Job drawing, mm, ordinate dimensions from the low corner. One solid piece. A direction names the side the tool comes from. Round coordinates to 2 decimals unless told otherwise and drop trailing zeros. Write each loop counter-clockwise with the first axis right and the second up, starting at its lowest first coordinate (ties: lowest second). Pieces come first, ordered by that corner, then holes. Notation, with made-up numbers: (47.25, 13) -> (52.25, 13) arc R23 ccw to (52.25, 42) -> close; hole circle Ø5 at (-2.75, -11). An arc over 180 degrees is marked (long way). Use CSV: the item, a comma, the result in double quotes. Start each with the question number.
(1) Saw through at B-B (x = 11). Give the cut face in (y, z), plus the area to 3 significant figures.
(2) Which spindle directions (+Z, -Z, +X, -X, +Y, -Y) get a long thin tool onto all of the face, cutting with end or side? Do the marked faces 1, 2 and 3. Say none if no direction does.
(3) Saw through at A-A (z = 5). Give the cut face in (x, y).
(4) Probe line 1 (Z direction, x = 11, y = 2.4); line 2 (X direction, y = 14.5, z = 4.75); line 3 (Y direction, x = 1.75, z = 4.75). List the from-to ranges inside material, lowest first. Write a range as [from, to].
(5) Saw through at D-D (x = 2.5). Give the cut face in (y, z).
(6) Drop flat-ended pins along their axis: pin 1 (2.5 mm diameter, centred on y = 11.5, z = 3.5, fed in from +X); pin 2 (3 mm diameter, centred on y = 15.5, z = 6.5, fed in from -X); pin 3 (1.5 mm diameter, centred on x = 18, z = 5.5, fed in from +Y); pin 4 (2.5 mm diameter, centred on y = 18.5, z = 7.5, fed in from +X). Give the stop position or say it passes through.
(7) Two-plate mould, pull along Y, no slides. Class the marked faces 4, 5 and 6: released by +Y, released by -Y, zero draft, split by the parting line, or undercut.
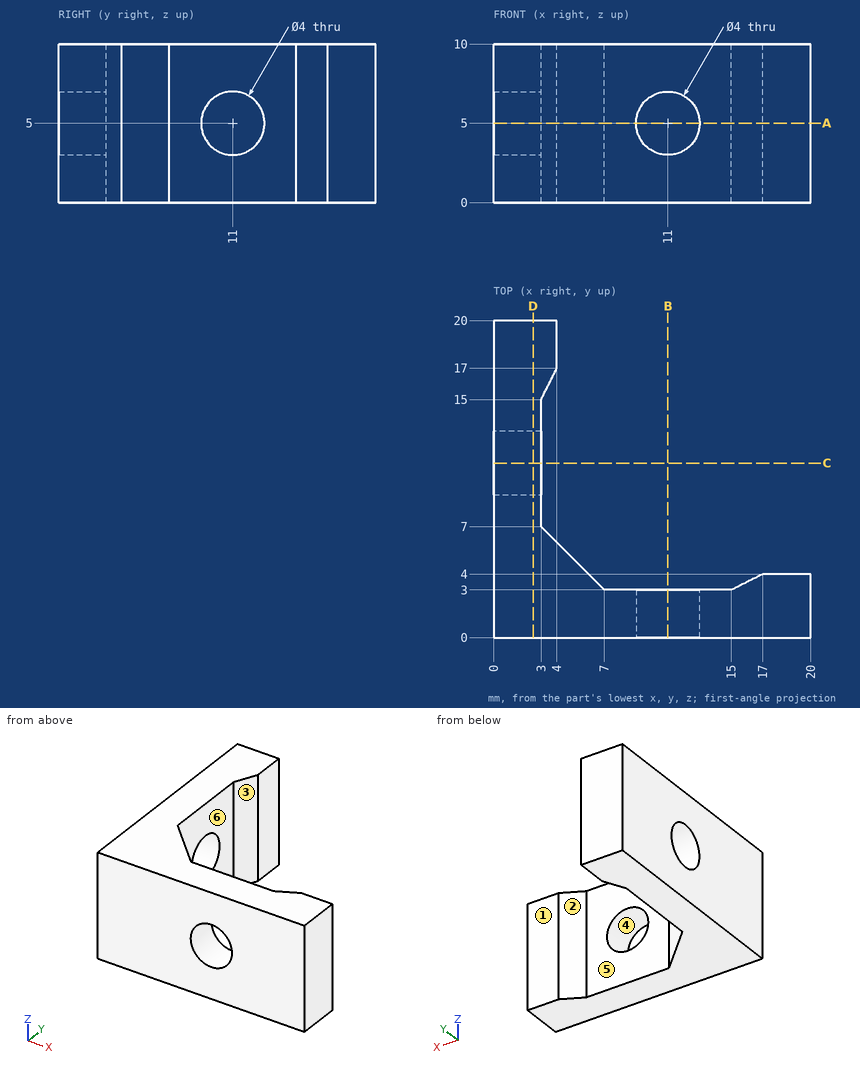
Answers:
1,outline,"(0, 0) -> (3, 0) -> (3, 3) -> (0, 3) -> close; (0, 7) -> (3, 7) -> (3, 10) -> (0, 10) -> close"
1,area,"18.0 mm²"
2,face 1,"+Z, -Z, +X, +Y"
2,face 2,"+Z, -Z, +Y"
2,face 3,"+Z, -Z, +X"
3,outline,"(0, 0) -> (9, 0) -> (9, 3) -> (7, 3) -> (3, 7) -> (3, 9) -> (0, 9) -> close; (0, 13) -> (3, 13) -> (3, 15) -> (4, 17) -> (4, 20) -> (0, 20) -> close; (13, 0) -> (20, 0) -> (20, 4) -> (17, 4) -> (15, 3) -> (13, 3) -> close"
4,line 1,"z = [0, 3], [7, 10]"
4,line 2,"x = [0, 3]"
4,line 3,"y = [0, 9.02], [12.98, 20]"
5,outline,"(0, 0) -> (20, 0) -> (20, 10) -> (0, 10) -> close; hole circle Ø4 at (11, 5)"
6,pin 1,"stops at x = 3"
6,pin 2,"stops at x = 0"
6,pin 3,"stops at y = 4"
6,pin 4,"stops at x = 4"
7,face 4,"zero draft"
7,face 5,"released by +Y"
7,face 6,"undercut"
